Could you check a few things on this model? Use its own coordinates, in mm. A direction names the side the tool comes from. Coordinates: 2 decimals unless noted, no trailing zeros. Order: outer loops, then holes, each group sorted by start corner. A loop starts at its lowest first (then second) coordinate and runs counter-clockwise, first axis right, second up. Notation, with made-up numbers: (43, -9.75) - (89, -9.75) arc R37 cw to (89, 27.25) - close; hole circle Ø7 at (43.25, -25). An arc over 180 degrees is marked (long way). Answer as a JSON object with one key per item and string values. Group by question number.
(1) We'd pull the mould along Z, two halves only. Please class faces 6 (the flat face through (176.276, 9, -38)), 7 (the cylindrical face through (56.53, 9.39, -70.18)), 8 (the flat face through (25, 9, -13.97)): pulls with the +Z half, pulls with the -Z half, needs draft (parallel to the pull), parting line crosses it, or undercut.
(2) Imagine slicing it at D-D, the plane x = 12. Write out the boundary of the cut face in (y, z).
(3) Which directions (+Z, -Z, +X, -X, +Y, -Y) give clear straight access to the entire face, cutting with the end or side of a thin tool? Please do faces 1 (the cylindrical face through (120.17, 9.39, -70.18)), 2 (the cylindrical face through (156.54, 9.6, -7.08)), 3 (the cylindrical face through (16.236, 10.479, -71.171)), 4 (the flat face through (22, 9, -77.61)), 5 (the flat face through (169.926, 9, -40)).
(4) Will these pins go through, and if not, where does the flat tip stop? P1, Ø4, axis at x = 102.5, y = 15, coming from the +Z side; P2, Ø8, axis at x = 124.5, z = -59.5, coming from the -Y side.
(5) Imagine slicing it at A-A, the plane x = 102.5. Write out the boundary of the cut face in (y, z), and give its area (3 significant figures).
(6) Imagine slicing it at B-B, the plane z = -39. Write out the boundary of the cut face in (x, y).
(7) Please list where these lines run through material, in increasing order: probe 1 along Z at (x, y) = (107, 1.25); probe 2 along X at (y, z) = (17.25, -19.5); probe 3 along X at (y, z) = (13.5, -11).
(8) Imagine slicing it at C-C, the plane y = 17.25. Write out the boundary of the cut face in (x, z), and give its area (3 significant figures).
from build123d import *

# Parameters (mm, degrees)
BOSS_EXTRUDE1_DEPTH            = 19.05
F_8_32_TAPPED_HOLE1_D          = 3.4544
F_8_32_TAPPED_HOLE1_DEPTH      = 13.97
F_10_CLEARANCE_HOLE1_D         = 5.1054
F_10_CLEARANCE_HOLE1_DEPTH     = 13.97
F_1_4_0_2500_DOWEL_HOLE2_D     = 6.35
F_1_4_0_2500_DOWEL_HOLE2_DEPTH = 12.7


with BuildPart() as part:
    # Sketch1 → Boss-Extrude1 (new body)
    with BuildSketch(Plane(origin=(0, 0, 0), x_dir=(1, 0, 0), z_dir=(0, 1, 0))):
        with BuildLine():
            Line((107.72869957, 77.6097), (68.54730043, 77.6097))
            ThreePointArc((68.54730043, 77.6097), (56.31815, 70.1802), (44.08899957, 77.6097))
            Line((44.08899957, 77.6097), (0, 77.6097))
            Line((0, 77.6097), (0, 0))
            Line((0, 0), (176.276, 0))
            Line((176.276, 0), (176.276, 77.6097))
            Line((176.276, 77.6097), (132.18700043, 77.6097))
            ThreePointArc((132.18700043, 77.6097), (119.95785, 70.1802), (107.72869957, 77.6097))
        make_face()
        with BuildLine():
            Line((169.926, 13.97), (132.18700043, 13.97))
            ThreePointArc((132.18700043, 13.97), (119.95785, 6.5405), (107.72869957, 13.97))
            Line((107.72869957, 13.97), (68.54730043, 13.97))
            ThreePointArc((68.54730043, 13.97), (56.31815, 6.5405), (44.08899957, 13.97))
            Line((44.08899957, 13.97), (6.35, 13.97))
            Line((6.35, 13.97), (6.35, 64.9097))
            Line((6.35, 64.9097), (169.926, 64.9097))
            Line((169.926, 64.9097), (169.926, 13.97))
        make_face(mode=Mode.SUBTRACT)
    extrude(amount=BOSS_EXTRUDE1_DEPTH)

    # #8-32 Tapped Hole1
    with Locations(Plane.XY):
        with Locations((154.813, 9.525), (21.463, 9.525)):
            Hole(F_8_32_TAPPED_HOLE1_D / 2, depth=F_8_32_TAPPED_HOLE1_DEPTH)

    # #10 Clearance Hole1
    with Locations(Plane.XY):
        with Locations((88.138, 9.525)):
            Hole(F_10_CLEARANCE_HOLE1_D / 2, depth=F_10_CLEARANCE_HOLE1_DEPTH)

    # 1/4 (0.2500) Dowel Hole2
    with Locations(Plane(origin=(0, 0, -77.6097), x_dir=(-1, 0, 0), z_dir=(0, 0, -1))):
        with Locations((-13.208, 9.525), (-163.068, 9.525)):
            Hole(F_1_4_0_2500_DOWEL_HOLE2_D / 2, depth=F_1_4_0_2500_DOWEL_HOLE2_DEPTH)


solid = part.part
Result set:
{
 "1": {"face 6": "needs draft", "face 7": "pulls with the -Z half", "face 8": "undercut"},
 "2": {"outline": "(0, -77.61) - (6.59, -77.61) - (6.59, -64.91) - (0, -64.91) - close; (0, -13.97) - (19.05, -13.97) - (19.05, 0) - (0, 0) - close; (12.46, -77.61) - (19.05, -77.61) - (19.05, -64.91) - (12.46, -64.91) - close"},
 "3": {"face 1": "-Z, +Y, -Y", "face 2": "+Z", "face 3": "-Z", "face 4": "-Z, +X, -X, +Y, -Y", "face 5": "+Y, -Y"},
 "4": {"P1": "stops at z = 0", "P2": "passes through"},
 "5": {"outline": "(0, -77.61) - (19.05, -77.61) - (19.05, -64.91) - (0, -64.91) - close; (0, -13.97) - (19.05, -13.97) - (19.05, 0) - (0, 0) - close", "area": "508 mm^2"},
 "6": {"outline": "(0, 0) - (6.35, 0) - (6.35, 19.05) - (0, 19.05) - close; (169.93, 0) - (176.28, 0) - (176.28, 19.05) - (169.93, 19.05) - close"},
 "7": {"probe 1": "z = -77.61 to -64.91, -13.97 to 0", "probe 2": "x = 0 to 6.35, 169.93 to 176.28", "probe 3": "x = 0 to 46.17, 66.47 to 109.81, 130.11 to 176.28"},
 "8": {"outline": "(0, -77.61) - (44.09, -77.61) arc R13.78 cw to (68.55, -77.61) - (107.73, -77.61) arc R13.78 cw to (132.19, -77.61) - (176.28, -77.61) - (176.28, 0) - (0, 0) - close; hole (6.35, -64.91) - (169.93, -64.91) - (169.93, -13.97) - (132.19, -13.97) arc R13.78 ccw to (107.73, -13.97) - (68.55, -13.97) arc R13.78 ccw to (44.09, -13.97) - (6.35, -13.97) - close", "area": "4,830 mm^2"}
}
